from build123d import *

# Parameters (mm, degrees)
SKETCH_R     = 40
SKETCH_R_2   = 10
PAD_DEPTH    = 10
SKETCH001_W  = 10
SKETCH001_H  = 30
PAD001_DEPTH = 20


with BuildPart() as part:
    # Sketch → Pad (new body)
    with BuildSketch(Plane.XY):
        Circle(SKETCH_R)
        Circle(SKETCH_R_2, mode=Mode.SUBTRACT)
    extrude(amount=PAD_DEPTH)

    # Sketch001 → Pad001 (new body)
    with BuildSketch(Plane.XY.offset(10)):
        with Locations((-27, 0)):
            Rectangle(SKETCH001_W, SKETCH001_H)
        with Locations((27, 0)):
            Rectangle(SKETCH001_W, SKETCH001_H)
    extrude(amount=PAD001_DEPTH)


solid = part.part
The listing builds one solid part. Answer for the finished solid, in the listing's coordinates (mm). A direction names the side the tool comes from. Give positions to 0.01 mm unless a question says otherwise; leave off trailing zeros. Write each loop counter-clockwise with the first axis right and the second up, starting at its lowest first coordinate (ties: lowest second). Pieces come first, ordered by that corner, then holes.
Item 1: Section B-B, the plane y = 0 is taken. Write down the section's boundary in (x, z), plus the area to 3 significant figures.
Item 2: Flat-ended cylindrical pins translate along their axes: P1, Ø10, axis at y = -5.5, z = 22, coming from the +X side; P2, Ø5, axis at x = -7.5, z = 9, coming from the +Y side; P3, Ø11, axis at x = 26.5, z = 24.5, coming from the -Y side. Find the tip coordinate at first contact, or state that the pin passes through.
Item 3: Which of the six approach directions +Z, -Z, +X, -X, +Y, -Y give full straight-line access (tool end or side, diameter ignored) to faces 1 (the flat face through (-27, -15, 20)), 2 (the flat face through (-27, 15, 20)), 3 (the flat face through (-22, 0, 20)), 4 (the flat face through (32, 0, 20))?
Item 4: Section C-C, the plane x = 0 is taken. Write down the section's boundary in (y, z), plus the area to 3 significant figures.
Item 5: Find the intervals of material crossed by line 1 along Y through (x, z) = (0, 2.5); line 2 along Z through (x, y) = (32.5, -8); line 3 along Y through (x, z) = (-29, 25.5), in increasing order.
Item 6: Determine the mould class of faces 5 (the flat face through (-32, 0, 20)), 6 (the cylindrical face through (-2.17, -9.76, 4.93)), 7 (the flat face through (27, 15, 20)) for opening direction X: released by +X, released by -X, zero draft, split by the parting line, or undercut.
Item 7: Section A-A, the plane z = 22 is taken. Write down the section's boundary in (x, y), plus the area to 3 significant figures.
Item 8: Section D-D, the plane z = 8.25 is taken. Write down the section's boundary in (x, y).
Completed:
1. outline: (-40, 0) - (-10, 0) - (-10, 10) - (-22, 10) - (-22, 30) - (-32, 30) - (-32, 10) - (-40, 10) - close; (10, 0) - (40, 0) - (40, 10) - (32, 10) - (32, 30) - (22, 30) - (22, 10) - (10, 10) - close
1. area: 1,000 mm2
2. P1: stops at x = 32
2. P2: stops at y = 39.69
2. P3: stops at y = -15
3. face 1: +Z, +X, -X, -Y
3. face 2: +Z, +X, -X, +Y
3. face 3: +Z, +Y, -Y
3. face 4: +Z, +X, +Y, -Y
4. outline: (-40, 0) - (-10, 0) - (-10, 10) - (-40, 10) - close; (10, 0) - (40, 0) - (40, 10) - (10, 10) - close
4. area: 600 mm2
5. line 1: y = -40 to -10, 10 to 40
5. line 2: z = 0 to 10
5. line 3: y = -15 to 15
6. face 5: released by -X
6. face 6: undercut
6. face 7: zero draft
7. outline: (-32, -15) - (-22, -15) - (-22, 15) - (-32, 15) - close; (22, -15) - (32, -15) - (32, 15) - (22, 15) - close
7. area: 600 mm2
8. outline: circle Ø80 at (0, 0); hole circle Ø20 at (0, 0)
